Build history of the part. All positions in model axes, mm. Face numbers are marked on the shaded views. A direction names the side the tool comes from. Round coordinates to 2 decimals unless told otherwise and drop trailing zeros. Loops run counter-clockwise (first coordinate to the right, second up) from the corner with the lowest first, then second, coordinate; pieces in that order, holes last. Notation, with made-up numbers: (-37.5, 59) - (-21.5, 59) arc R30 ccw to (-21.5, 91) - close; hole circle Ø2 at (80, -5). An arc over 180 degrees is marked (long way). One line per question, with ' | ' between items. Start each with the question number.
from build123d import *

# Parameters (mm, degrees)
F0_R     = 5
F1_DEPTH = 3
F3_DEPTH = 6


with BuildPart() as f1:
    # F0 (on Top) → F1 (new body)
    with BuildSketch(Plane.XY):
        with BuildLine():
            ThreePointArc((20, 10), (17.071068, 17.071068), (10, 20))
            Line((10, 20), (-10, 20))
            ThreePointArc((-10, 20), (-17.071068, 17.071068), (-20, 10))
            Line((-20, 10), (-20, -10))
            ThreePointArc((-20, -10), (-17.071068, -17.071068), (-10, -20))
            Line((-10, -20), (10, -20))
            ThreePointArc((10, -20), (17.071068, -17.071068), (20, -10))
            Line((20, -10), (20, 10))
        make_face()
        Circle(F0_R, mode=Mode.SUBTRACT)
    extrude(amount=F1_DEPTH)

    # F2 (on face) → F3 (join)
    with BuildSketch(Plane.XY.offset(3)):
        with BuildLine():
            ThreePointArc((17, 10), (14.949747, 14.949747), (10, 17))
            Line((10, 17), (-10, 17))
            ThreePointArc((-10, 17), (-14.949747, 14.949747), (-17, 10))
            Line((-17, 10), (-17, -10))
            ThreePointArc((-17, -10), (-14.949747, -14.949747), (-10, -17))
            Line((-10, -17), (10, -17))
            ThreePointArc((10, -17), (14.949747, -14.949747), (17, -10))
            Line((17, -10), (17, 10))
        make_face()
        with BuildLine():
            Line((-10, 15.5), (10, 15.5))
            ThreePointArc((10, 15.5), (13.889087, 13.889087), (15.5, 10))
            Line((15.5, 10), (15.5, -10))
            ThreePointArc((15.5, -10), (13.889087, -13.889087), (10, -15.5))
            Line((10, -15.5), (-10, -15.5))
            ThreePointArc((-10, -15.5), (-13.889087, -13.889087), (-15.5, -10))
            Line((-15.5, -10), (-15.5, 10))
            ThreePointArc((-15.5, 10), (-13.889087, 13.889087), (-10, 15.5))
        make_face(mode=Mode.SUBTRACT)
    extrude(amount=F3_DEPTH)


solid = f1.part
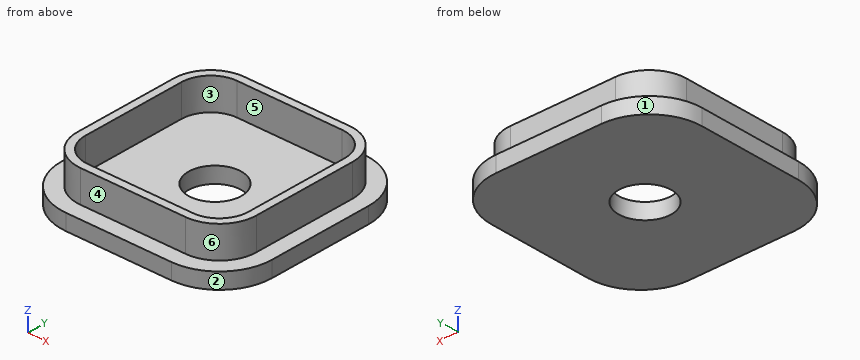
1) Saw through at D-D on y = -6.5. Write the cut outline in (x, z).
2) Drop flat-ended pins along their axis: pin 1 (1.8 mm diameter, centred on x = -2.5, z = 6.5, fed in from +Y); pin 2 (2 mm diameter, centred on x = -7, y = 13.5, fed in from -Z); pin 3 (2 mm diameter, centred on y = 7, z = 6, fed in from +X); pin 4 (5 mm diameter, centred on y = 11.5, z = 8, fed in from -X). Give the stop position or say it passes through.
3) Tool access for the marked faces 4, 5 and 6: list every direction of +Z, -Z, +X, -X, +Y, -Y with a clear straight run to the whole face (end or side of a thin tool).
4) Saw through at A-A on y = 0. Write the cut outline in (x, z), and give its area (3 significant figures).
5) Saw through at B-B on z = 2. Write the cut outline in (x, y), and give its area (3 significant figures).
6) Two-plate mould, pull along Y, no slides. Class the marked faces 1, 2 and 3: +Y half, -Y half, draft (parallel to the pull), parting line (faces both ways), or undercut.
7) Wall check: line 1 (Y direction, x = -5, z = 7.25); line 2 (Y direction, x = 0, z = 2.25). Give the ranges that are in metal, low to high. Write a range as [from, to].
Answer key:
1) outline: (-20, 0) - (20, 0) - (20, 3) - (17, 3) - (17, 9) - (15.5, 9) - (15.5, 3) - (-15.5, 3) - (-15.5, 9) - (-17, 9) - (-17, 3) - (-20, 3) - close
2) pin 1: y = 17 | pin 2: z = 0 | pin 3: x = 17 | pin 4: x = -17
3) face 4: +Z, +X, -X, -Y | face 5: +Z | face 6: +Z, +X, -Y
4) outline: (-20, 0) - (-5, 0) - (-5, 3) - (-15.5, 3) - (-15.5, 9) - (-17, 9) - (-17, 3) - (-20, 3) - close; (5, 0) - (20, 0) - (20, 3) - (17, 3) - (17, 9) - (15.5, 9) - (15.5, 3) - (5, 3) - close | area: 108 mm²
5) outline: (-20, -10) arc R10 ccw to (-10, -20) - (10, -20) arc R10 ccw to (20, -10) - (20, 10) arc R10 ccw to (10, 20) - (-10, 20) arc R10 ccw to (-20, 10) - close; hole circle Ø10 at (0, 0) | area: 1,440 mm²
6) face 1: +Y half | face 2: -Y half | face 3: undercut
7) line 1: [-17, -15.5], [15.5, 17] | line 2: [-20, -5], [5, 20]
